from build123d import *

# Parameters (mm, degrees)
F1_DEPTH = 25
F2_R     = 1.5
F3_R     = 1.99999


# Not quite as in the source:
# - a fillet or chamfer is up to 0.001 mm smaller than in the source, because OpenCascade refuses the exact size


with BuildPart() as f1:
    # F0 (on Top) → F1 (new body)
    with BuildSketch(Plane.XY):
        Polygon((24.5, 0), (0, 0), (0, -37), (2, -37), (2, -2), (22.5, -2), (22.5, -12), (24.5, -12), align=None)
    extrude(amount=F1_DEPTH)

    # F2
    f2_edges = [f1.edges().sort_by_distance(p)[0] for p in [
        (22.5, -12, 12.5),
    ]]
    fillet(f2_edges, radius=F2_R)

    # F3 (radius 2 in the source; OpenCascade refuses exactly that, so slightly less here)
    f3_edges = [f1.edges().sort_by_distance(p)[0] for p in [
        (0, 0, 12.5),
        (0, -37, 12.5),
    ]]
    fillet(f3_edges, radius=F3_R)


solid = f1.part
Source: CAD feature listing. Evaluate the final solid. Frame: model axes, mm. A direction names the side the tool comes from. Round coordinates to 2 decimals unless told otherwise and drop trailing zeros. Order: outer loops, then holes, each group sorted by start corner. A loop starts at its lowest first (then second) coordinate and runs counter-clockwise, first axis right, second up. Notation, with made-up numbers: (38, -23) -> (49, -23) arc R25 ccw to (49, -8) -> close; hole circle Ø8 at (-4, 20). An arc over 180 degrees is marked (long way). Answer as CSV lines item,"result".
Item 1: Section A-A, the plane y = -9.5. Return loops of the section in (x, z).
A:
outline,"(0, 0) -> (2, 0) -> (2, 25) -> (0, 25) -> close; (22.5, 0) -> (24.5, 0) -> (24.5, 25) -> (22.5, 25) -> close"
Item 2: Pin query (flat end, axial travel): pin 1 Ø4 at (x, z) = (21, 21) entering from -Y; pin 2 Ø4 at (x, z) = (6.5, 6) entering from -Y; pin 3 Ø0.6 at (x, z) = (24.5, 17.5) entering from -Y. Return the tip coordinate at first contact, or that it passes through.
A:
pin 1,"y = -11.62"
pin 2,"y = -2"
pin 3,"y = -12"
Item 3: Line query: L1, parallel to X at y = -5, z = 20.25; L2, parallel to X at y = -22.5, z = 19.25; L3, parallel to Y at x = 8, z = 7.75. Output: solid intervals per line, ascending.
A:
L1,"0 to 2, 22.5 to 24.5"
L2,"0 to 2"
L3,"-2 to 0"
Item 4: Section C-C, the plane x = 3.5. Return loops of the section in (y, z), plus the area to 3 significant figures.
A:
outline,"(-2, 0) -> (0, 0) -> (0, 25) -> (-2, 25) -> close"
area,"50.0 mm²"
Item 5: Section D-D, the plane y = -20. Return loops of the section in (x, z).
A:
outline,"(0, 0) -> (2, 0) -> (2, 25) -> (0, 25) -> close"
Item 6: Reachability of faces 1 (the face through (12, -2, 12)), 2 (the face through (24.5, -6, 12)) from +Z, -Z, +X, -X, +Y, -Y: full face, straight path, thin tool, end or side. Return the list, or none.
A:
face 1,"+Z, -Z, -Y"
face 2,"+Z, -Z, +X, +Y, -Y"
